Part print with two shaded views. Sizes in mm from the minimum x, y, z corner. A direction names the side the tool comes from. Round coordinates to 2 decimals unless told otherwise and drop trailing zeros. Write each loop counter-clockwise with the first axis right and the second up, starting at its lowest first coordinate (ties: lowest second). Pieces come first, ordered by that corner, then holes.
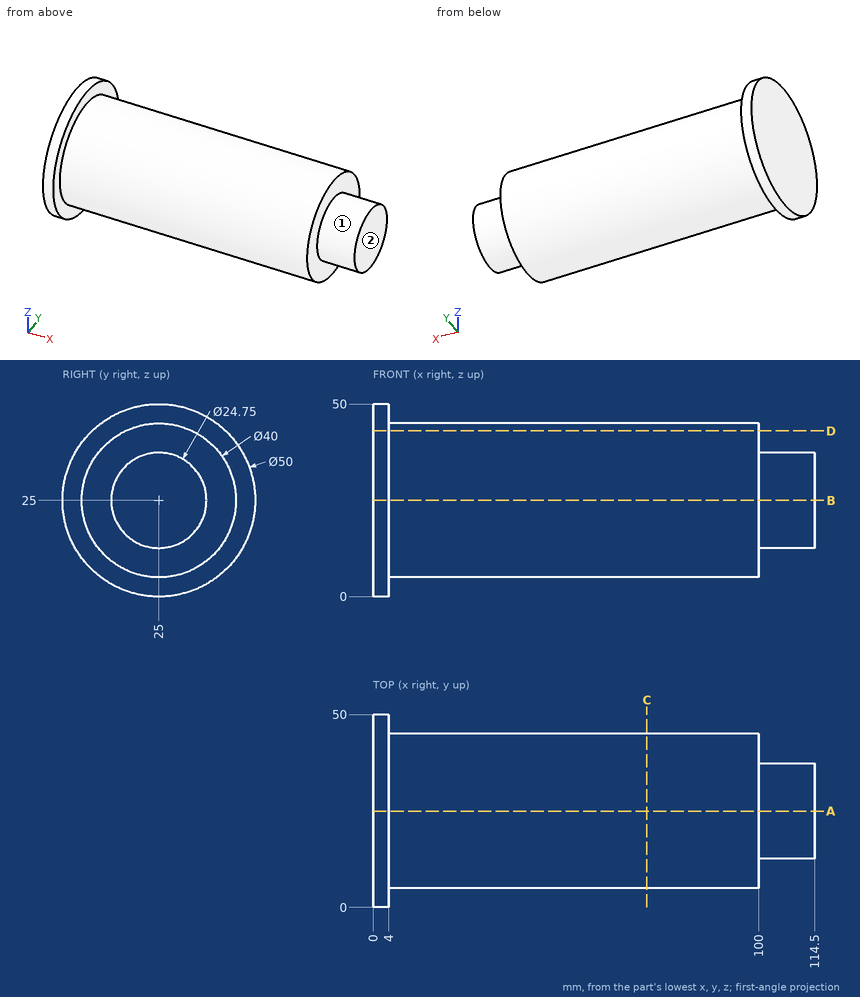
Q1. Which spindle directions (+Z, -Z, +X, -X, +Y, -Y) get a long thin tool onto all of the face, cutting with end or side? Do the marked faces 1 and 2. Say none if no direction does.
Values follow:
face 1: +X
face 2: +Z, -Z, +X, +Y, -Y
Q2. Wall check: L1, parallel to X at y = 33, z = 41; L2, parallel to X at y = 21, z = 4; L3, parallel to Z at x = 81, y = 24.5. Give the ranges that are in metal, low to high.
Values follow:
L1: x = 0 to 100
L2: x = 0 to 4
L3: z = 5.01 to 44.99
Q3. Drop flat-ended pins along their axis: pin 1 (10 mm diameter, centred on x = 81, y = 39.5, fed in from +Z); pin 2 (1.5 mm diameter, centred on y = 30.5, z = 6, fed in from +X); pin 3 (1 mm diameter, centred on y = 5.5, z = 15.5, fed in from +X). Give the stop position or say it passes through.
Values follow:
pin 1: stops at z = 42.6
pin 2: stops at x = 100
pin 3: stops at x = 4
Q4. Cut at A-A on y = 25. Write the cut outline in (x, z) (3 decimals), plus the area to 3 significant figures.
Values follow:
outline: (0, 0) - (4, 0) - (4, 5) - (100, 5) - (100, 12.625) - (114.5, 12.625) - (114.5, 37.375) - (100, 37.375) - (100, 45) - (4, 45) - (4, 50) - (0, 50) - close
area: 4,400 mm2
Q5. Cut at D-D on z = 43. Write the cut outline in (x, y).
Values follow:
outline: (0, 7.65) - (4, 7.65) - (4, 16.28) - (100, 16.28) - (100, 33.72) - (4, 33.72) - (4, 42.35) - (0, 42.35) - close
Q6. Cut at C-C on x = 71. Write the cut outline in (y, z).
Values follow:
outline: circle Ø40 at (25, 25)
